Work out the finished part from the listing and answer in its coordinate system (mm). Round coordinates to 2 decimals unless told otherwise and drop trailing zeros. Write each loop counter-clockwise with the first axis right and the second up, starting at its lowest first coordinate (ties: lowest second). Pieces come first, ordered by that corner, then holes. Notation, with made-up numbers: (45, -29) -> (86, -29) arc R24 ccw to (86, 10) -> close; hole circle Ø1 at (2.25, 2). An arc over 180 degrees is marked (long way). One line per item, written item: value.
Solid Edge part; units mm, degrees
sketch "Sketch1" plane through (0, 0, 0) normal (0, 0, 1) x (1, 0, 0)
  circle A0 centre (0, 15) radius 7.5
  circle A1 centre (0, -10) radius 7.5
  line L0 (25, 25) -> (-25, 25)
  line L1 (-25, 25) -> (-25, -25)
  line L2 (-25, -25) -> (25, -25)
  line L3 (25, -25) -> (25, 25)
  dimension "D1" = 25
  dimension "D2" = 25
extrude "Protrusion1" add sketch "Sketch1" along normal blind 10
(1) Consider probe 1 along Y at (x, z) = (0, 3); probe 2 along Y at (x, z) = (-1, 5); probe 3 along X at (y, z) = (16, 1). Determine where each line is inside the solid, lowest interval first.
Reported:
probe 1: y = -25 to -17.5, -2.5 to 7.5, 22.5 to 25
probe 2: y = -25 to -17.43, -2.57 to 7.57, 22.43 to 25
probe 3: x = -25 to -7.43, 7.43 to 25
(2) Find section D-D on y = -8.5. Give the vertices of the cut face in (x, z), plus the area to 3 significant figures.
Reported:
outline: (-25, 0) -> (-7.35, 0) -> (-7.35, 10) -> (-25, 10) -> close; (7.35, 0) -> (25, 0) -> (25, 10) -> (7.35, 10) -> close
area: 353 mm2
(3) For a pull along Y with two mould halves and no side action, classify faces 1 (the face through (0, 25, 5)), 2 (the face through (-1.63, -2.68, 4.93)), 3 (the face through (-25, 0, 5)) as pulls with the +Y half, pulls with the -Y half, needs draft (parallel to the pull), parting line crosses it, or undercut.
Reported:
face 1: pulls with the +Y half
face 2: undercut
face 3: needs draft
(4) Find section C-C on z = 4. Give the vertices of the cut face in (x, y), plus the area to 3 significant figures.
Reported:
outline: (-25, -25) -> (25, -25) -> (25, 25) -> (-25, 25) -> close; hole circle Ø15 at (0, -10); hole circle Ø15 at (0, 15)
area: 2,150 mm2
(5) Find section B-B on x = 0. Give the vertices of the cut face in (y, z), plus the area to 3 significant figures.
Reported:
outline: (-25, 0) -> (-17.5, 0) -> (-17.5, 10) -> (-25, 10) -> close; (-2.5, 0) -> (7.5, 0) -> (7.5, 10) -> (-2.5, 10) -> close; (22.5, 0) -> (25, 0) -> (25, 10) -> (22.5, 10) -> close
area: 200 mm2
(6) Find section A-A on y = 15. Give the vertices of the cut face in (x, z).
Reported:
outline: (-25, 0) -> (-7.5, 0) -> (-7.5, 10) -> (-25, 10) -> close; (7.5, 0) -> (25, 0) -> (25, 10) -> (7.5, 10) -> close
(7) A flat-ended cylindrical pin translates along its axis: pin 1 Ø13.5 at (x, y) = (0, -10) entering from +Z. Find the tip coordinate at first contact, or state that the pin passes through.
Reported:
pin 1: passes through
